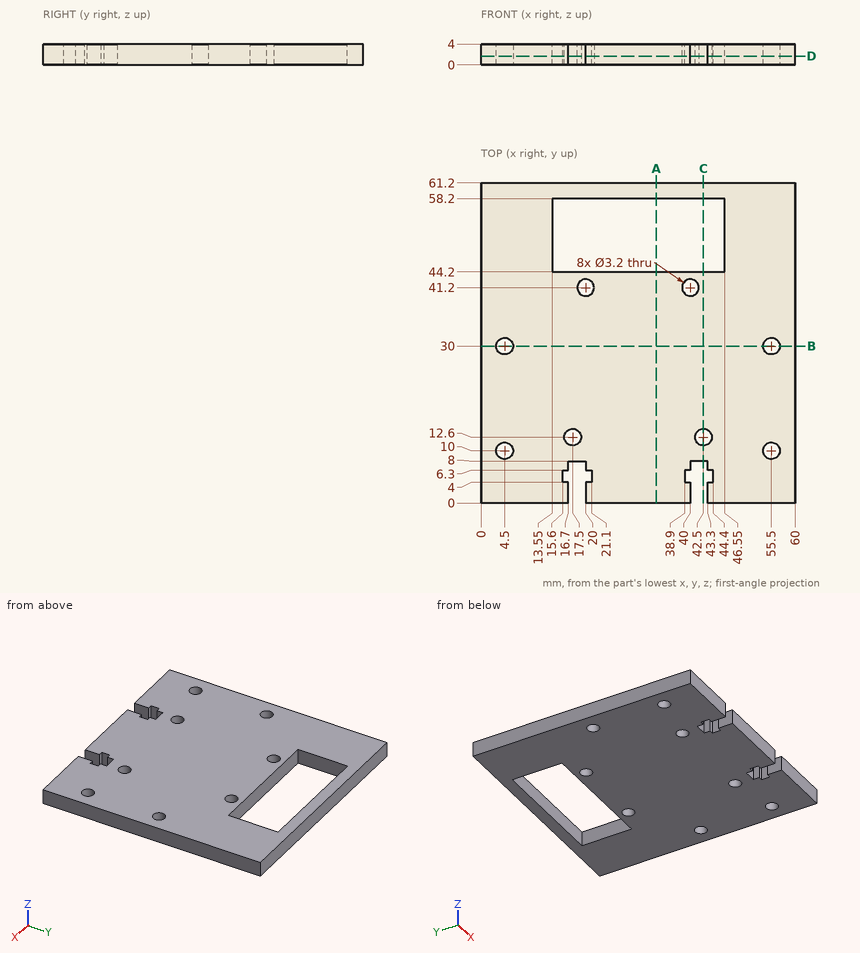
The drawing under review shows one solid part. Ordinate dimensions are in mm from its lowest x, y, z. Round coordinates to 2 decimals unless told otherwise and drop trailing zeros. Loops run counter-clockwise (first coordinate to the right, second up) from the corner with the lowest first, then second, coordinate; pieces in that order, holes last. Notation, with made-up numbers: M 61.25,4 L 111.25,4 A25 cw 111.25,43 Z; hole C -25.75,-4.5 d1. An arc over 180 degrees is marked long. Answer as CSV lines item,"result". Start each with the question number.
Item 1: Consider section D-D (z = 1.7). State how many separate pieces and enclosed holes the cut face has, then the cut area to 3 significant figures.
Item 2: Consider section B-B (y = 30). Write out the cut boundary in (x, z), then the cut area to 3 significant figures.
Item 3: Consider section C-C (x = 42.5). Write out the cut boundary in (y, z), then the cut area to 3 significant figures.
Item 4: Consider section A-A (x = 33.5). Write out the cut boundary in (y, z).
Item 5: Wall thickness on line 1 (Y direction, x = 55.5, z = 2.3); line 2 (Y direction, x = 46.5, z = 3.7); line 3 (X direction, y = 31, z = 1): over which ranges is each line inside the solid? List them lowest first. Write a range as [from, to].
Answer:
1,separate pieces,"1"
1,enclosed holes,"9"
1,area,"3,080 mm^2"
2,outline,"M 0,0 L 2.9,0 L 2.9,4 L 0,4 Z; M 6.1,0 L 53.9,0 L 53.9,4 L 6.1,4 Z; M 57.1,0 L 60,0 L 60,4 L 57.1,4 Z"
2,area,"214 mm^2"
3,outline,"M 8,0 L 11,0 L 11,4 L 8,4 Z; M 14.2,0 L 44.2,0 L 44.2,4 L 14.2,4 Z; M 58.2,0 L 61.2,0 L 61.2,4 L 58.2,4 Z"
3,area,"144 mm^2"
4,outline,"M 0,0 L 44.2,0 L 44.2,4 L 0,4 Z; M 58.2,0 L 61.2,0 L 61.2,4 L 58.2,4 Z"
5,line 1,"y = [0, 8.4], [11.6, 28.4], [31.6, 61.2]"
5,line 2,"y = [0, 44.2], [58.2, 61.2]"
5,line 3,"x = [0, 3.25], [5.75, 54.25], [56.75, 60]"
